Design review of the part built by this model. Coordinates are the model's own, in mm. Face numbers are marked on the shaded views. A direction names the side the tool comes from. Round coordinates to 2 decimals unless told otherwise and drop trailing zeros. Write each loop counter-clockwise with the first axis right and the second up, starting at its lowest first coordinate (ties: lowest second). Pieces come first, ordered by that corner, then holes. Notation, with made-up numbers: (-1.5, 49) -> (41.5, 49) arc R13 ccw to (41.5, 74) -> close; hole circle Ø3 at (59.5, 87.25). An arc over 180 degrees is marked (long way). Write item = value, one per line. Start each with the question number.
Item 1: Add section B-B, the plane z = 30. State the section outline as (x, y) points, then the cut area to 3 significant figures.
Item 2: For pin 1 Ø9 at (x, z) = (46, 6) entering from +Y; pin 2 Ø1 at (x, z) = (-12, 6) entering from -Y; pin 3 Ø12 at (y, z) = (15, 38.5) entering from -X; pin 4 Ø5 at (x, z) = (46, 30) entering from -Y, all flat-tipped, find the tip position at first contact; note any pin that passes through.
Item 3: Add section C-C, the plane y = 16. State the section outline as (x, z) points.
Item 4: Add section A-A, the plane x = 46. State the section outline as (y, z) points.
Item 5: Add section D-D, the plane z = 39. State the section outline as (x, y) points.
Item 6: Machinability: for the marked faces 1, 2 and 3, which of the approach directions +Z, -Z, +X, -X, +Y, -Y give a long, thin tool a straight path to every point of the face, cutting with its end or side? Answer none if there is none.
Item 7: To check wall thickness, follow L1, parallel to Z at x = 46, y = 15; L2, parallel to X at y = 16, z = 16; L3, parallel to Y at x = 47.5, z = 8.5. State the ranges of each line that lie inside material, in increasing order.
from build123d import *

# Parameters (mm, degrees)
CYLINDER001_R          = 2.75
CYLINDER001_DEPTH      = 15
CYLINDER001_ROLL_ANGLE = 90
CYLINDER002_R          = 2.75
CYLINDER002_DEPTH      = 15
CYLINDER002_ROLL_ANGLE = 90
CYLINDER003_R          = 2.75
CYLINDER003_DEPTH      = 15
CYLINDER003_ROLL_ANGLE = 90
CYLINDER_R             = 2.75
CYLINDER_DEPTH         = 15
CYLINDER_ROLL_ANGLE    = 90
BOX_W                  = 20
BOX_H                  = 11
BOX_DEPTH              = 52
BOX001_W               = 10
BOX001_H               = 31
BOX001_DEPTH           = 52
CYLINDER004_R          = 35
CYLINDER004_DEPTH      = 52


with BuildPart() as cylinder001:
    # Cylinder001 → Cylinder001 (new body)
    with BuildSketch(Plane.XY):
        Circle(CYLINDER001_R)
    extrude(amount=CYLINDER001_DEPTH)


with BuildPart() as cylinder001_1:
    # Cylinder001 roll: moved
    add(cylinder001.part.rotate(Axis((0, 0, 0), (1, 0, 0)), CYLINDER001_ROLL_ANGLE))


with BuildPart() as cylinder001_2:
    # Cylinder001 placement: moved
    add(cylinder001_1.part.moved(Location((46, 23, 6))))


with BuildPart() as cylinder002:
    # Cylinder002 → Cylinder002 (new body)
    with BuildSketch(Plane.XY):
        Circle(CYLINDER002_R)
    extrude(amount=CYLINDER002_DEPTH)


with BuildPart() as cylinder002_1:
    # Cylinder002 roll: moved
    add(cylinder002.part.rotate(Axis((0, 0, 0), (1, 0, 0)), CYLINDER002_ROLL_ANGLE))


with BuildPart() as cylinder002_2:
    # Cylinder002 placement: moved
    add(cylinder002_1.part.moved(Location((46, 23, 16))))


with BuildPart() as cylinder003:
    # Cylinder003 → Cylinder003 (new body)
    with BuildSketch(Plane.XY):
        Circle(CYLINDER003_R)
    extrude(amount=CYLINDER003_DEPTH)


with BuildPart() as cylinder003_1:
    # Cylinder003 roll: moved
    add(cylinder003.part.rotate(Axis((0, 0, 0), (1, 0, 0)), CYLINDER003_ROLL_ANGLE))


with BuildPart() as cylinder003_2:
    # Cylinder003 placement: moved
    add(cylinder003_1.part.moved(Location((46, 23, 45))))


with BuildPart() as negative_fusion:
    # Cylinder → Cylinder (new body)
    with BuildSketch(Plane.XY):
        Circle(CYLINDER_R)
    extrude(amount=CYLINDER_DEPTH)


with BuildPart() as negative_fusion_1:
    # Cylinder roll: moved
    add(negative_fusion.part.rotate(Axis((0, 0, 0), (1, 0, 0)), CYLINDER_ROLL_ANGLE))


with BuildPart() as negative_fusion_2:
    # Cylinder placement: moved
    add(negative_fusion_1.part.moved(Location((46, 23, 30))))

    # Fusion: union Cylinder001, Cylinder002, Cylinder003
    add(cylinder001_2.part)
    add(cylinder002_2.part)
    add(cylinder003_2.part)


with BuildPart() as cube:
    # Box → Box (new body)
    with BuildSketch(Plane(origin=(36, 10, 0), x_dir=(1, 0, 0), z_dir=(0, 0, 1))):
        with Locations((10, 5.5)):
            Rectangle(BOX_W, BOX_H)
    extrude(amount=BOX_DEPTH)


with BuildPart() as cube001:
    # Box001 → Box001 (new body)
    with BuildSketch(Plane(origin=(26, -10, 0), x_dir=(1, 0, 0), z_dir=(0, 0, 1))):
        with Locations((5, 15.5)):
            Rectangle(BOX001_W, BOX001_H)
    extrude(amount=BOX001_DEPTH)


with BuildPart() as cut:
    # Cylinder004 → Cylinder004 (new body)
    with BuildSketch(Plane.XY):
        Circle(CYLINDER004_R)
    extrude(amount=CYLINDER004_DEPTH)

    # Fusion001: union Cube, Cube001
    add(cube.part)
    add(cube001.part)

    # Cut: cut Negative Fusion
    add(negative_fusion_2.part, mode=Mode.SUBTRACT)


solid = cut.part
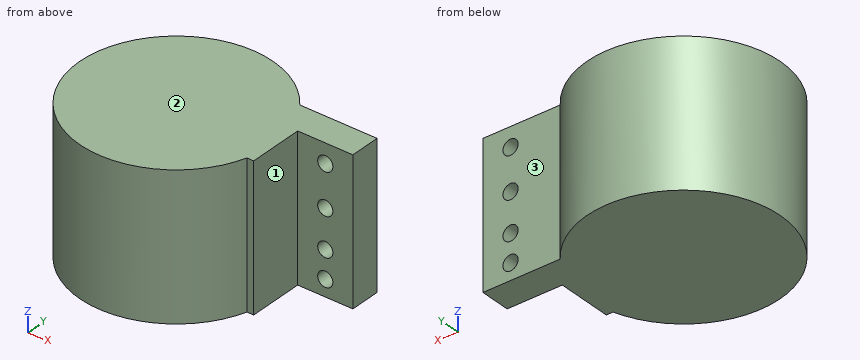
Result set:
q1.outline = (28, 21) arc R35 ccw (long way) to (33.54, -10) -> (36, -10) -> (36, 10) -> (43.25, 10) -> (43.25, 21) -> close; (48.75, 10) -> (56, 10) -> (56, 21) -> (48.75, 21) -> close
q1.area = 4,090 mm²
q2.pin_1 = 21
q2.pin_2 = -33.06
q2.pin_3 = -33.82
q2.pin_4 = through
q3.outline = (-31.13, 0) -> (56, 0) -> (56, 52) -> (-31.13, 52) -> close; hole circle Ø5.5 at (46, 6); hole circle Ø5.5 at (46, 16); hole circle Ø5.5 at (46, 30); hole circle Ø5.5 at (46, 45)
q4.outline = (10, 0) -> (21, 0) -> (21, 3.25) -> (10, 3.25) -> close; (10, 8.75) -> (21, 8.75) -> (21, 13.25) -> (10, 13.25) -> close; (10, 18.75) -> (21, 18.75) -> (21, 27.25) -> (10, 27.25) -> close; (10, 32.75) -> (21, 32.75) -> (21, 42.25) -> (10, 42.25) -> close; (10, 47.75) -> (21, 47.75) -> (21, 52) -> (10, 52) -> close
q5.outline = (28, 21) arc R35 ccw (long way) to (33.54, -10) -> (36, -10) -> (36, 10) -> (56, 10) -> (56, 21) -> close
q6.face_1 = +Z, -Z, +X, -Y
q6.face_2 = +Z, +X, -X, +Y, -Y
q6.face_3 = +Z, -Z, +X, +Y
q7.L1 = 0 to 3.25, 8.75 to 13.25, 18.75 to 27.25, 32.75 to 42.25, 47.75 to 52
q7.L2 = -31.13 to 43.25, 48.75 to 56
q7.L3 = 10 to 21
